Drawing for the job (mm, zero at the part's lowest x, y, z). A direction names the side the tool comes from. Give positions to 0.01 mm unless a question says otherwise; leave off trailing zeros. Loops run counter-clockwise (first coordinate to the right, second up) from the corner with the lowest first, then second, coordinate; pieces in that order, holes last. Notation, with made-up numbers: (25, 77.5) -> (41, 77.5) arc R30 cw to (41, 99.5) -> close; hole circle Ø8 at (-31.75, 51.5). An arc over 180 degrees is marked (long way). Write item = value, one per line.
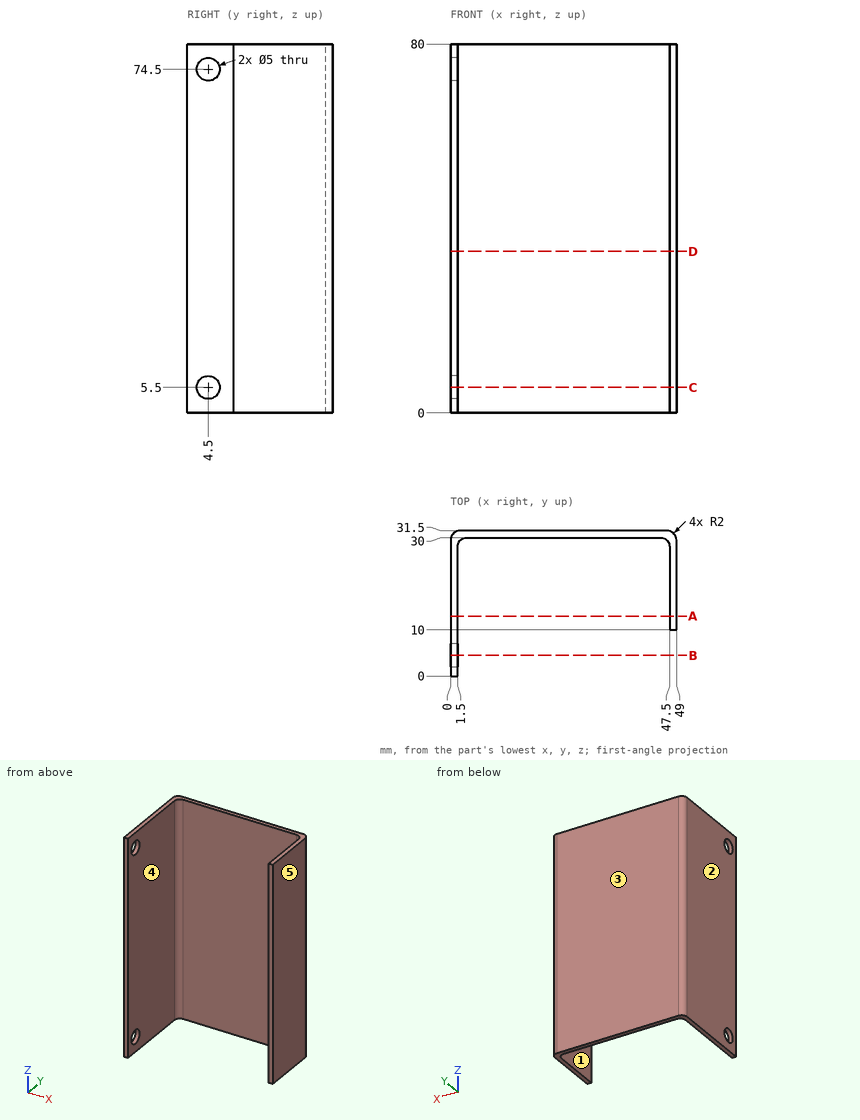
1) Slice it at B-B, the plane y = 4.5. List the corners of the cut face in (x, z).
Resolved:
outline = (0, 0) -> (1.5, 0) -> (1.5, 3) -> (0, 3) -> close; (0, 8) -> (1.5, 8) -> (1.5, 72) -> (0, 72) -> close; (0, 77) -> (1.5, 77) -> (1.5, 80) -> (0, 80) -> close
2) Pull direction X, two halves, no side cores. Call the marked faces 1, 2 and 3: pulls with the +X half, pulls with the -X half, needs draft (parallel to the pull), parting line crosses it, or undercut.
Resolved:
face_1 = undercut
face_2 = pulls with the -X half
face_3 = needs draft
3) Slice it at D-D, the plane z = 35. List the corners of the cut face in (x, y), and give its area (4 significant figures).
Resolved:
outline = (0, 0) -> (1.5, 0) -> (1.5, 28) arc R2 cw to (3.5, 30) -> (45.5, 30) arc R2 cw to (47.5, 28) -> (47.5, 10) -> (49, 10) -> (49, 29.5) arc R2 ccw to (47, 31.5) -> (2, 31.5) arc R2 ccw to (0, 29.5) -> close
area = 148.5 mm²
4) Slice it at C-C, the plane z = 5.5. List the corners of the cut face in (x, y), and give its area (3 significant figures).
Resolved:
outline = (0, 0) -> (1.5, 0) -> (1.5, 2) -> (0, 2) -> close; (0, 7) -> (1.5, 7) -> (1.5, 28) arc R2 cw to (3.5, 30) -> (45.5, 30) arc R2 cw to (47.5, 28) -> (47.5, 10) -> (49, 10) -> (49, 29.5) arc R2 ccw to (47, 31.5) -> (2, 31.5) arc R2 ccw to (0, 29.5) -> close
area = 141 mm²
5) Drop flat-ended pins along their axis: P1, Ø8, axis at y = 4.5, z = 74.5, coming from the +X side; P2, Ø1.6, axis at x = 48, z = 40.5, coming from the -Y side; P3, Ø12.5, axis at x = 29, z = 32.5, coming from the -Y side. Give the stop position or say it passes through.
Resolved:
P1 = 1.5
P2 = 10
P3 = 30
6) Which spindle directions (+Z, -Z, +X, -X, +Y, -Y) get a long thin tool onto all of the face, cutting with end or side? Do the marked faces 4 and 5. Say none if no direction does.
Resolved:
face_4 = +Z, -Z, -Y
face_5 = +Z, -Z, +X, +Y, -Y
7) Slice it at A-A, the plane y = 13. List the corners of the cut face in (x, z).
Resolved:
outline = (0, 0) -> (1.5, 0) -> (1.5, 80) -> (0, 80) -> close; (47.5, 0) -> (49, 0) -> (49, 80) -> (47.5, 80) -> close
8) Drill centre lines: line 1 along Z through (x, y) = (0.6, 4.5); line 2 along X through (y, z) = (14.5, 33); line 3 along X through (y, z) = (3.5, 58.5). Where is each one in solid material? Low to high. Write a range as [from, to].
Resolved:
line_1 = [0, 3], [8, 72], [77, 80]
line_2 = [0, 1.5], [47.5, 49]
line_3 = [0, 1.5]
